Source: CAD feature listing. Evaluate the final solid. Frame: model axes, mm. Round coordinates to 2 decimals unless told otherwise and drop trailing zeros. Order: outer loops, then holes, each group sorted by start corner. A loop starts at its lowest first (then second) coordinate and runs counter-clockwise, first axis right, second up. Notation, with made-up numbers: (5.25, 30.25) - (49.25, 30.25) arc R25 ccw to (49.25, 62.25) - close; hole circle Ø9 at (78, -1.5). An arc over 180 degrees is marked (long way). Use one line per item in the form item = value. Start each with the question number.
Q1. Cut plane A-A, the plane y = 0. Return the cut outline in (x, z), and give its area (3 significant figures).
Q2. Ray query, line 1 (Z direction, x = 0.8, y = 0); line 2 (Y direction, x = 0.75, z = 15); line 3 (Y direction, x = 0.4, z = -30.5). Return the intervals inside material, ascending. Write a range as [from, to].
Q3. Cut plane D-D, the plane x = 1.65. Give the number of separate pieces and of enclosed holes in the cut face, and give its area (3 significant figures).
Q4. Cut plane C-C, the plane y = -18.5. Return the cut outline in (x, z).
Q5. Cut plane B-B, the plane z = 22.5. Return the cut outline in (x, y).
Q6. Pin query (flat end, axial travel): pin 1 Ø1.5 at (x, z) = (1, -3) entering from -Y; pin 2 Ø1.5 at (x, y) = (1, 42) entering from +Z; pin 3 Ø10 at (y, z) = (17.5, 17.5) entering from +X; pin 4 Ø0.9 at (x, y) = (1.5, -12.5) entering from -Z. Return the tip coordinate at first contact, or that it passes through.
Autodesk Inventor part; units mm, degrees
ref_plane "YZ Plane" through (0, 0, 0) normal (1, 0, 0) x (0, 1, 0)
ref_plane "XZ Plane" through (0, 0, 0) normal (0, 1, 0) x (-1, 0, 0)
ref_plane "XY Plane" through (0, 0, 0) normal (0, 0, 1) x (1, 0, 0)
sketch "Sketch1" plane through (0, 0, 0) normal (1, 0, 0) x (0, 1, 0)
  line L0 (-40.7216, -13) -> (-2, -13)
  arc A0 (30.5631, 9.4815) -> (-30.5631, 9.4815) centre (0, 0) ccw
  arc A1 (8.4591, 5.3333) -> (-8.4591, 5.3333) centre (0, 0) ccw
  circle A2 centre (0, 0) radius 1.5
  line L1 (3, -18) -> (3, -43.0842)
  arc A3 (3, -18) -> (-2, -13) centre (-2, -18) ccw
  arc A4 (6.4138, -46.0555) -> (-45.6278, -8.9639) centre (0, 0) ccw
  line L2 (-12.6886, 3) -> (-25.7876, 3)
  line L3 (12.6886, 3) -> (25.7876, 3)
  arc A5 (-30.5631, 9.4815) -> (-25.7876, 3) centre (-25.7876, 8) ccw
  arc A6 (-12.6886, 3) -> (-8.4591, 5.3333) centre (-12.6886, 8) ccw
  arc A7 (8.4591, 5.3333) -> (12.6886, 3) centre (12.6886, 8) ccw
  arc A8 (25.7876, 3) -> (30.5631, 9.4815) centre (25.7876, 8) ccw
  arc A9 (-45.6278, -8.9639) -> (-40.7216, -13) centre (-40.7216, -8) ccw
  arc A10 (3, -43.0842) -> (6.4138, -46.0555) centre (6, -43.0842) ccw
  point P0 (-44.6458, -13)
  point P1 (3, -13)
  point P2 (-10, 0)
  point P3 (10, 0)
  point P4 (-9.5394, 3)
  point P5 (9.5394, 3)
  point P6 (3, -31.881)
  point P7 (3, -46.4031)
  point P8 (-31.8591, 3)
  point P9 (31.8591, 3)
  dimension "d5" = 32
  dimension "d6" = 20
  dimension "d7" = 3
  dimension "d52" = 3
  dimension "d53" = 3
  dimension "d54" = 5
  dimension "d66" = 46.5
  dimension "d78" = 16
  dimension "d79" = 5
  dimension "d80" = 3
  dimension "d81" = 3
  dimension "d82" = 5
extrude "Extrusion3" add sketch "Sketch1" along normal blind 3
sketch "Sketch2" plane through (3, 0, 0) normal (1, 0, 0) x (0, 0, -1)
  arc A0 (-9.4815, 30.5631) -> (-9.4815, -30.5631) centre (0, 0) ccw
  line L0 (8, 43) -> (13, 43)
  line L1 (13, 43) -> (13, 40)
  line L2 (13, 40) -> (8, 40)
  line L3 (8, 40) -> (8, 43)
  dimension "d38" = 3
  dimension "d41" = 40
  dimension "d42" = 8
  dimension "d43" = 5
extrude "Extrusion5" cut sketch "Sketch2" against normal through all
sketch "Sketch4" plane through (3, 0, 0) normal (1, 0, 0) x (0, 0, -1)
  arc A0 (-9.4815, 30.5631) -> (-9.4815, -30.5631) centre (0, 0) ccw
  line L0 (-3, 25.7876) -> (-3, 12.6886)
  line L1 (-3, -12.6886) -> (-3, -25.7876)
  line L2 (-3, -20) -> (6, -20)
  line L3 (6, -20) -> (6, -25)
  line L4 (6, -25) -> (-3, -25)
  line L5 (-3, -25) -> (-3, -20)
  line L6 (-3, 17.5) -> (6, 17.5)
  line L7 (6, 17.5) -> (6, 12.5)
  line L8 (6, 12.5) -> (-3, 12.5)
  line L9 (-3, 12.5) -> (-3, 17.5)
  dimension "d57" = 9
  dimension "d59" = 5
  dimension "d60" = 20
  dimension "d61" = 9
  dimension "d62" = 5
  dimension "d63" = 12.5
extrude "Extrusion6" cut sketch "Sketch4" against normal through all
sketch "Sketch5" plane through (3, 0, 0) normal (1, 0, 0) x (0, 0, -1)
  line L0 (-3, 17.5) -> (0, 17.5)
  line L1 (0, 17.5) -> (0, 22.5)
  line L2 (0, 22.5) -> (-3, 22.5)
  line L3 (-3, 22.5) -> (-3, 17.5)
  point P0 (0, 0)
  dimension "d67" = 5
  dimension "d68" = 3
extrude "Extrusion7" cut sketch "Sketch5" against normal through all
sketch "Sketch6" plane through (3, 0, 0) normal (1, 0, 0) x (0, 0, -1)
  circle A0 centre (0, 0) radius 1.5
  arc A1 (32.8695, 15.8696) -> (21.1594, 29.741) centre (0, 0) ccw
  line L0 (31.0685, 13) -> (20, 13)
  line L1 (18, 15) -> (18, 28.1114)
  line L2 (18, 3) -> (43.0842, 3)
  line L3 (13, -40.7216) -> (13, -2)
  arc A2 (31.0685, 13) -> (32.8695, 15.8696) centre (31.0685, 15) ccw
  arc A3 (21.1594, 29.741) -> (18, 28.1114) centre (20, 28.1114) ccw
  arc A4 (18, 15) -> (20, 13) centre (20, 15) ccw
  point P0 (41.1696, 0.4856)
  point P1 (14.881, -40.3065)
  point P2 (14.881, -4.5144)
  point P3 (18, 31.753)
  point P4 (34.1065, 13)
  point P5 (43.0842, 3)
  point P6 (13, -2)
  dimension "d72" = 73
  dimension "d73" = 10
  dimension "d74" = 5
  dimension "d75" = 2
extrude "Extrusion8" cut sketch "Sketch6" against normal through all contours A2 L0 A4 L1 A3 A1
properties part number "EChasisSide2"
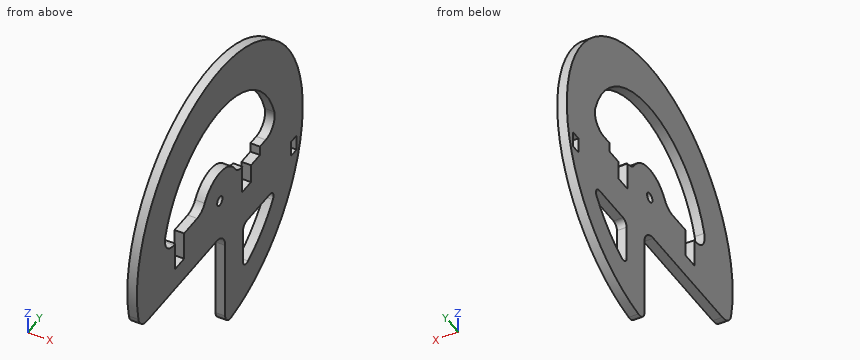
Completed:
q1.outline = (0, -13.42) - (3, -13.42) - (3, -1.5) - (0, -1.5) - close; (0, 1.5) - (3, 1.5) - (3, 10) - (0, 10) - close; (0, 32) - (3, 32) - (3, 46.5) - (0, 46.5) - close
q1.area = 105 mm2
q2.line_1 = [-13.42, -1.5], [1.5, 10], [32, 46.5]
q2.line_2 = [-44.01, -28.27], [28.27, 44.01]
q2.line_3 = [3, 13], [20.05, 35.1]
q3.separate_pieces = 1
q3.enclosed_holes = 4
q3.area = 3,990 mm2
q4.outline = (0, -13) - (3, -13) - (3, 3) - (0, 3) - close; (0, 26.11) - (3, 26.11) - (3, 42.66) - (0, 42.66) - close
q5.outline = (0, -40.69) - (3, -40.69) - (3, -22.75) - (0, -22.75) - close; (0, 22.75) - (3, 22.75) - (3, 40.69) - (0, 40.69) - close
q6.pin_1 = -46.45
q6.pin_2 = 21.46
q6.pin_3 = through
q6.pin_4 = -13
